Geometry: see drawing. Coordinates: mm, zero at the bounding-box minimum. A direction names the side the tool comes from. Round coordinates to 2 decimals unless told otherwise and drop trailing zeros. Loops run counter-clockwise (first coordinate to the right, second up) from the corner with the lowest first, then second, coordinate; pieces in that order, holes last. Notation, with made-up numbers: (1.5, -7.75) -> (58.5, -7.75) arc R24 cw to (58.5, 6.25) -> close; hole circle Ø9 at (-2.75, 13). An arc over 180 degrees is marked (long way). Answer in a Markdown table with one row per item.
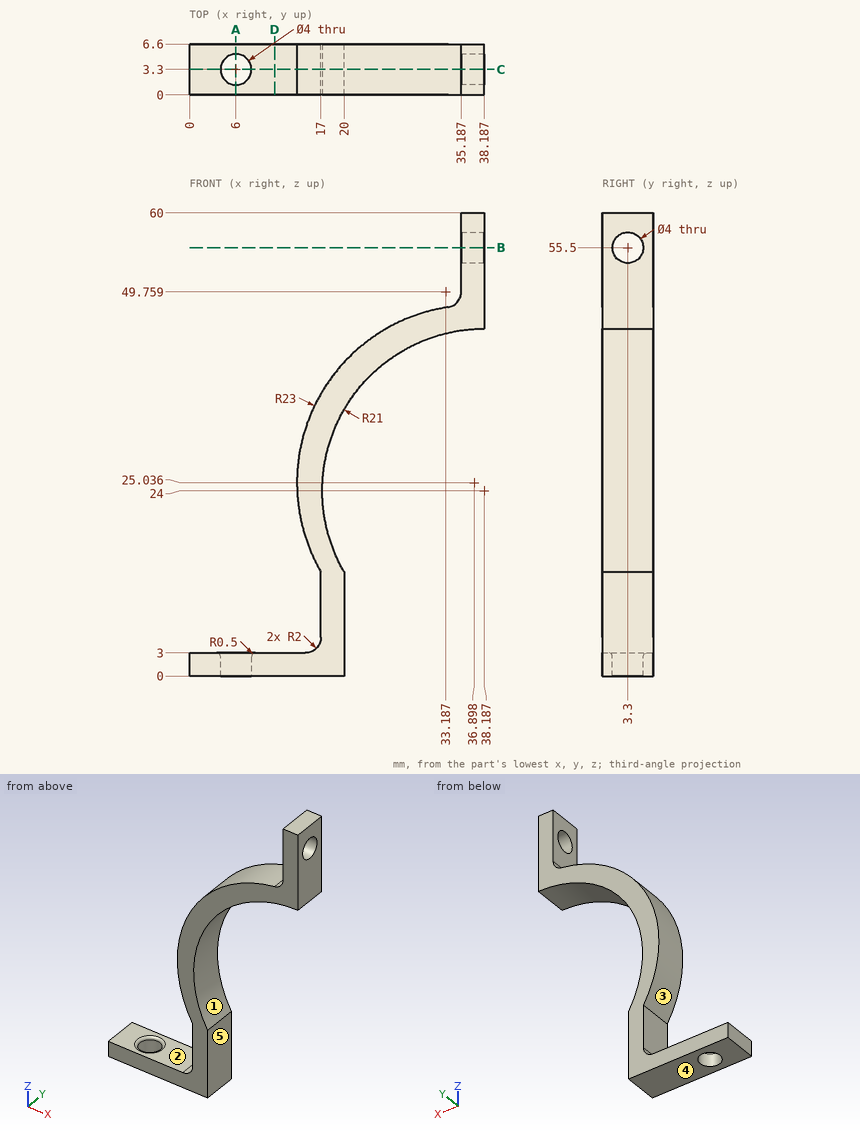
Item 1: Set-up query: the marked faces 1 and 2. Return all of +Z, -Z, +X, -X, +Y, -Y with unobstructed straight access to the full face (end or side cutting, diameter ignored); none if empty.
Ans:
| item | result |
|---|---|
| face 1 | +X, +Y, -Y |
| face 2 | -X, +Y, -Y |
Item 2: First-contact query: P1, Ø1.5, axis at x = 27, y = 5.5, coming from the -Z side; P2, Ø3.5, axis at x = 9, y = 2, coming from the +Z side. Flat tips, straight axial feed; report the tip coordinate or a pass-through.
Ans:
| item | result |
|---|---|
| P1 | z = 41.28 |
| P2 | z = 3 |
Item 3: Section query D-D, the plane x = 11. Output: boundary loops of the cut face in (y, z), and give its area (3 significant figures).
Ans:
| item | result |
|---|---|
| outline | (0, 0) -> (6.6, 0) -> (6.6, 3) -> (0, 3) -> close |
| area | 19.8 mm2 |
Item 4: Section query A-A, the plane x = 6. Output: boundary loops of the cut face in (y, z).
Ans:
| item | result |
|---|---|
| outline | (0, 0) -> (1.3, 0) -> (1.3, 2.5) arc R0.5 ccw to (0.8, 3) -> (0, 3) -> close; (5.3, 0) -> (6.6, 0) -> (6.6, 3) -> (5.8, 3) arc R0.5 ccw to (5.3, 2.5) -> close |
Item 5: Section query C-C, the plane y = 3.3. Output: boundary loops of the cut face in (x, z), and give its area (3 significant figures).
Ans:
| item | result |
|---|---|
| outline | (0, 0) -> (4, 0) -> (4, 2.5) arc R0.5 ccw to (3.5, 3) -> (0, 3) -> close; (8, 0) -> (20, 0) -> (20, 13.5) arc R21 cw to (38.19, 45) -> (38.19, 53.5) -> (35.19, 53.5) -> (35.19, 49.76) arc R2 cw to (33.48, 47.78) arc R23 ccw to (17, 13.5) -> (17, 5) arc R2 cw to (15, 3) -> (8.5, 3) arc R0.5 ccw to (8, 2.5) -> close; (35.19, 57.5) -> (38.19, 57.5) -> (38.19, 60) -> (35.19, 60) -> close |
| area | 261 mm2 |
Item 6: Ray query, L1, parallel to Y at x = 6, z = 0.85; L2, parallel to X at y = 6.5, z = 56.5; L3, parallel to Z at x = 12.5, y = 1.5. Return the intervals inside material, ascending.
Ans:
| item | result |
|---|---|
| L1 | 0 to 1.3, 5.3 to 6.6 |
| L2 | 35.19 to 38.19 |
| L3 | 0 to 3 |
Item 7: Section query B-B, the plane z = 55.5. Output: boundary loops of the cut face in (x, y).
Ans:
| item | result |
|---|---|
| outline | (35.19, 0) -> (38.19, 0) -> (38.19, 1.3) -> (35.19, 1.3) -> close; (35.19, 5.3) -> (38.19, 5.3) -> (38.19, 6.6) -> (35.19, 6.6) -> close |
Item 8: Mould query, pull axis Z, two halves, no side actions, for the marked faces 3, 4 and 5. Classes: released by +Z, released by -Z, zero draft, split by the parting line, or undercut.
Ans:
| item | result |
|---|---|
| face 3 | undercut |
| face 4 | released by -Z |
| face 5 | zero draft |
